For this review, take the finished solid that the model builds, in its own axes (mm). A direction names the side the tool comes from. Round coordinates to 2 decimals unless told otherwise and drop trailing zeros. Write each loop counter-clockwise with the first axis right and the second up, starting at its lowest first coordinate (ties: lowest second). Pieces come first, ordered by that corner, then holes. Notation, with made-up numbers: (17.5, -24.5) -> (49.5, -24.5) arc R20 cw to (49.5, 3.5) -> close; hole circle Ø4 at (22.5, 10). An arc over 180 degrees is marked (long way). Write item = value, one per line. Start each with the question number.
Autodesk Inventor part; units mm, degrees
ref_plane "YZ Plane" through (0, 0, 0) normal (1, 0, 0) x (0, 1, 0)
ref_plane "XZ Plane" through (0, 0, 0) normal (0, 1, 0) x (-1, 0, 0)
ref_plane "XY Plane" through (0, 0, 0) normal (0, 0, 1) x (1, 0, 0)
sketch "Skizze1" plane through (0, 0, 0) normal (0, 0, 1) x (1, 0, 0)
  line L0 (-14.5, -16.5) -> (14.5, -16.5)
  line L1 (14.5, -16.5) -> (14.5, 16.5)
  line L2 (14.5, 16.5) -> (-14.5, 16.5)
  line L3 (-14.5, 16.5) -> (-14.5, -16.5)
  point P0 (0, 0)
  point P1 (-14.5, 0)
  point P2 (0, -16.5)
  dimension "d0" = 29
  dimension "d1" = 33
extrude "Extrusion1" add sketch "Skizze1" along normal blind 6
hole "Hole1" at (-10, 12.5, 6) direction (0, 0, -1) diameter 3 end through all
pattern_linear "Rechteckige Anordnung1" count 2 spacing 20 along (1, 0, 0) of "Hole1"
sketch "Skizze2" plane through (0, 0, 6) normal (0, 0, 1) x (1, 0, 0)
  circle A0 centre (-10, 12.5) radius 3
  line L0 (14.5, -16.5) -> (-14.5, -16.5)
  line L1 (-14.5, 16.5) -> (14.5, 16.5)
  line L2 (0, 16.5) -> (0, -16.5)
  circle A1 centre (10, 12.5) radius 1.5
  point P0 (0, 0)
  point P1 (0, -11.2)
  dimension "d42" = 23.7
hole "Hole2" at (0, -11.2, 6) at (-10, 12.5, 6) direction (0, 0, -1) diameter 3 end through all
sketch "Skizze3" plane through (0, 0, 0) normal (0, 0, -1) x (-1, 0, 0)
  line L0 (14.5, -16.5) -> (-14.5, -16.5)
  line L1 (-14.5, 16.5) -> (14.5, 16.5)
  line L2 (0, -16.5) -> (0, 16.5)
  point P0 (0, 0)
  point P1 (0, 10.7)
  dimension "d24" = 5.8
hole "Hole3" at (0, 10.7, 0) direction (0, 0, 1) diameter 4 end through all
sketch "Skizze4" plane through (0, 0, 0) normal (0, 0, -1) x (-1, 0, 0)
  circle A0 centre (0, 10.7) radius 2
  line L0 (0, 6.6585) -> (-3.5, 8.6793)
  line L1 (-3.5, 8.6793) -> (-3.5, 12.7207)
  line L2 (-3.5, 12.7207) -> (0, 14.7415)
  line L3 (0, 14.7415) -> (3.5, 12.7207)
  line L4 (3.5, 12.7207) -> (3.5, 8.6793)
  line L5 (3.5, 8.6793) -> (0, 6.6585)
  point P0 (0, 0)
  dimension "d32" = 7
extrude "Extrusion2" cut sketch "Skizze4" against normal blind 3.3
sketch "Skizze5" plane through (0, 0, 6) normal (0, 0, 1) x (1, 0, 0)
  line L0 (-14.5, -16.5) -> (-14.5, 16.5)
  line L1 (14.5, -16.5) -> (-14.5, -16.5)
  line L2 (-14.5, 16.5) -> (14.5, 16.5)
  line L3 (-14.5, 8.5) -> (-6, 4.5)
  line L4 (-6, 4.5) -> (-6, -16.5)
  line L5 (0, 16.5) -> (0, -16.5)
  line L6 (14.5, -16.5) -> (14.5, 16.5)
  line L7 (-14.5, -16.5) -> (14.5, -16.5)
  line L8 (14.5, 8.5) -> (6, 4.5)
  line L9 (6, 4.5) -> (6, -16.5)
  point P0 (0, 0)
  dimension "d36" = 12
  dimension "d37" = 8
  dimension "d38" = 6
extrude "Extrusion3" cut sketch "Skizze5" against normal blind 6 contours L0 L3 L4 L1 | L9 L8 L6 L1
fillet "Rundung1" radius 2 8 edges at (6, 4.5, 3) (6, -16.5, 3) (-6, -16.5, 3) (-6, 4.5, 3) (-14.5, 8.5, 3) (-14.5, 16.5, 3) (14.5, 16.5, 3) (14.5, 8.5, 3)
properties part number "adapterplatte"
1. Clearance check with flat-ended pins moving along their axes: pin 1 Ø1.8 at (y, z) = (-9, 4) entering from -X; pin 2 Ø1.8 at (y, z) = (-9, 2) entering from +X; pin 3 Ø3.5 at (x, y) = (-1, 11) entering from -Z. State where each tip first meets the part, or that it passes through.
2. Wall thickness on L1, parallel to X at y = 12.5, z = 3.15; L2, parallel to Y at x = 0, z = 2.5; L3, parallel to X at y = 12.5, z = 3.5: over which ranges is each line inside the solid? List them lowest first. Write a range as from..to.
3. Machinability: for faces 1 (the flat face through (3.5, 11, 2)), 2 (the flat face through (6, -6, 3)), 3 (the flat face through (14.5, 12, 3)), which of the approach directions +Z, -Z, +X, -X, +Y, -Y give a long, thin tool a straight path to every point of the face, cutting with its end or side? Answer none if there is none.
4. Consider section A-A, the plane z = 4.95. Give the boundary of the cut face in (x, y).
5. Draft analysis for pull direction Y (two halves, no side actions). For faces 4 (the cylindrical face through (-6.32, 4.316, 2.958)), 5 (the flat face through (-6, -6, 3)), 6 (the cylindrical face through (-9.1, 13.7, 3)), 7 (the flat face through (1.726, 7.655, 1.627)), state which applies: +Y half, -Y half, draft (parallel to the pull), parting line (faces both ways), or undercut.
6. Consider section B-B, the plane y = -11.2. Give the boundary of the cut face in (x, z), then the cut area to 3 significant figures.
7. Consider section D-D, the plane z = 1. Give the boundary of the cut face in (x, y).
8. Consider section C-C, the plane x = 0.75. Give the boundary of the cut face in (y, z).
Outcome:
q1.pin_1 = -6
q1.pin_2 = 6
q1.pin_3 = 3.3
q2.L1 = -14.5..-11.5, -8.5..-3.5, 3.5..8.5, 11.5..14.5
q2.L2 = -16.5..-12.7, -9.7..6.66, 14.74..16.5
q2.L3 = -14.5..-11.5, -8.5..-0.87, 0.87..8.5, 11.5..14.5
q3.face_1 = -Z
q3.face_2 = +Z, -Z, +X, -Y
q3.face_3 = +Z, -Z, +X, +Y, -Y
q4.outline = (-14.5, 9.77) arc R2 ccw to (-13.35, 7.96) -> (-7.15, 5.04) arc R2 cw to (-6, 3.23) -> (-6, -14.5) arc R2 ccw to (-4, -16.5) -> (4, -16.5) arc R2 ccw to (6, -14.5) -> (6, 3.23) arc R2 cw to (7.15, 5.04) -> (13.35, 7.96) arc R2 ccw to (14.5, 9.77) -> (14.5, 14.5) arc R2 ccw to (12.5, 16.5) -> (-12.5, 16.5) arc R2 ccw to (-14.5, 14.5) -> close; hole circle Ø3 at (-10, 12.5); hole circle Ø4 at (0, 10.7); hole circle Ø3 at (0, -11.2); hole circle Ø3 at (10, 12.5)
q5.face_4 = -Y half
q5.face_5 = draft
q5.face_6 = undercut
q5.face_7 = undercut
q6.outline = (-6, 0) -> (-1.5, 0) -> (-1.5, 6) -> (-6, 6) -> close; (1.5, 0) -> (6, 0) -> (6, 6) -> (1.5, 6) -> close
q6.area = 54.0 mm2
q7.outline = (-14.5, 9.77) arc R2 ccw to (-13.35, 7.96) -> (-7.15, 5.04) arc R2 cw to (-6, 3.23) -> (-6, -14.5) arc R2 ccw to (-4, -16.5) -> (4, -16.5) arc R2 ccw to (6, -14.5) -> (6, 3.23) arc R2 cw to (7.15, 5.04) -> (13.35, 7.96) arc R2 ccw to (14.5, 9.77) -> (14.5, 14.5) arc R2 ccw to (12.5, 16.5) -> (-12.5, 16.5) arc R2 ccw to (-14.5, 14.5) -> close; hole circle Ø3 at (-10, 12.5); hole (-3.5, 8.68) -> (0, 6.66) -> (3.5, 8.68) -> (3.5, 12.72) -> (0, 14.74) -> (-3.5, 12.72) -> close; hole circle Ø3 at (0, -11.2); hole circle Ø3 at (10, 12.5)
q8.outline = (-16.5, 0) -> (-12.5, 0) -> (-12.5, 6) -> (-16.5, 6) -> close; (-9.9, 0) -> (7.09, 0) -> (7.09, 3.3) -> (8.85, 3.3) -> (8.85, 6) -> (-9.9, 6) -> close; (12.55, 3.3) -> (14.31, 3.3) -> (14.31, 0) -> (16.5, 0) -> (16.5, 6) -> (12.55, 6) -> close
